```python
from build123d import *

# Parameters (mm, degrees)
RESSALTO_EXTRUS_O1_DEPTH   = 10
ESBO_O2_W                  = 6
ESBO_O2_H                  = 2.5
RESSALTO_EXTRUS_O2_DEPTH   = 8
ESBO_O3_W                  = 2.8
ESBO_O3_H                  = 2.8
CORTE_EXTRUS_O1_DEPTH      = 25.104680044
ESBO_O4_W                  = 6
ESBO_O4_H                  = 18
ESBO_O4_W_2                = 2.8
ESBO_O4_H_2                = 2.8
RESSALTO_EXTRUS_O3_DEPTH   = 2
CORTE_EXTRUS_O3_DEPTH      = 23.633727046
CORTE_EXTRUS_O3_DEPTH_BACK = 23.633727046
CORTE_EXTRUS_O4_DEPTH      = 24.796756081


with BuildPart() as part:
    # Esboço1 → Ressalto-extrusão1 (new body)
    with BuildSketch(Plane.XY):
        Polygon((-0.4, 0), (-0.57, 0), (-0.57, -2.5), (5.43, -2.5), (5.43, 0), (5.26, 0), (5.26, 10), (5.66, 11.25), (5.24, 12.5), (4.44, 12.5), (4.04, 11.25), (4.44, 10), (4.44, 0), (2.84, 0), (2.84, 10), (3.24, 11.25), (2.82, 12.5), (2.02, 12.5), (1.62, 11.25), (2.02, 10), (2.02, 0), (0.42, 0), (0.42, 10), (0.82, 11.25), (0.4, 12.5), (-0.4, 12.5), (-0.8, 11.25), (-0.4, 10), align=None)
    extrude(amount=RESSALTO_EXTRUS_O1_DEPTH)

    # Esboço2 → Ressalto-extrusão2 (add)
    with BuildSketch(Plane.XY.offset(10)):
        with Locations((2.43, -1.25)):
            Rectangle(ESBO_O2_W, ESBO_O2_H)
    extrude(amount=RESSALTO_EXTRUS_O2_DEPTH)

    # Esboço3 → Corte-extrusão1 (cut, through all)
    with BuildSketch(Plane.XZ.offset(2.5)):
        with Locations((2.43, 14)):
            Rectangle(ESBO_O3_W, ESBO_O3_H)
    extrude(amount=-CORTE_EXTRUS_O1_DEPTH, mode=Mode.SUBTRACT)

    # Esboço4 → Ressalto-extrusão3 (add)
    with BuildSketch(Plane.XZ.offset(2.5)):
        with Locations((2.43, 9)):
            Rectangle(ESBO_O4_W, ESBO_O4_H)
        with Locations((2.43, 14)):
            Rectangle(ESBO_O4_W_2, ESBO_O4_H_2, mode=Mode.SUBTRACT)
    extrude(amount=RESSALTO_EXTRUS_O3_DEPTH)

    # Esboço6 → Corte-extrusão3 (cut, two sides: drawn at the far end of the back side and taken through both)
    with BuildSketch(Plane(origin=(0, 0, 0), x_dir=(0, 0, -1), z_dir=(1, 0, 0)).offset(-CORTE_EXTRUS_O3_DEPTH_BACK)):
        Polygon((-18, 0), (-18, -2), (-14, -2), (-10.8, -2), (-10, 0), align=None)
    extrude(amount=CORTE_EXTRUS_O3_DEPTH + CORTE_EXTRUS_O3_DEPTH_BACK, mode=Mode.SUBTRACT)

    # Esboço7 → Corte-extrusão4 (cut, through all)
    with BuildSketch(Plane(origin=(0, -2, 0), x_dir=(1, 0, 0), z_dir=(0, 1, 0))):
        with BuildLine():
            Line((-0.57, -15.5), (-3.321312229, -15.5))
            Line((-3.321312229, -15.5), (-3.321312229, -18.857639181))
            Line((-3.321312229, -18.857639181), (8.546861735, -18.857639181))
            Line((8.546861735, -18.857639181), (8.546861735, -15.5))
            Line((8.546861735, -15.5), (5.43, -15.5))
            ThreePointArc((5.43, -15.5), (4.697766953, -17.267766953), (2.93, -18))
            Line((2.93, -18), (1.93, -18))
            ThreePointArc((1.93, -18), (0.162233047, -17.267766953), (-0.57, -15.5))
        make_face()
    extrude(amount=-CORTE_EXTRUS_O4_DEPTH, mode=Mode.SUBTRACT)


solid = part.part
```
The model under review builds one solid part; all positions refer to its coordinate system, in mm. A direction names the side the tool comes from. Round coordinates to 2 decimals unless told otherwise and drop trailing zeros. Loops run counter-clockwise (first coordinate to the right, second up) from the corner with the lowest first, then second, coordinate; pieces in that order, holes last. Notation, with made-up numbers: (40.5, 66.5) - (53.5, 66.5) arc R31 cw to (53.5, 101.5) - close; hole circle Ø1 at (64, -10). An arc over 180 degrees is marked (long way). Write each question's results on one line, items separated by ' | '. Start each with the question number.
Q1. Insertion check: P1, Ø3, axis at y = 8, z = 7.5, coming from the +X side; P2, Ø3, axis at y = -3.5, z = 14.5, coming from the +X side; P3, Ø3.5, axis at y = -2, z = 4, coming from the -X side; P4, Ø3, axis at x = 2.5, y = -3.5, coming from the -Z side. Each pin has a flat end and moves straight along its axis. Give the tip position at first contact, or say it passes through.
Q2. Take a section at A-A on z = 13.75. Give the boundary of the cut face in (x, y).
Q3. Wall thickness on line 1 along X through (y, z) = (6.5, 9.5); line 2 along X through (y, z) = (12.25, 4.5); line 3 along Z through (x, y) = (2.5, -2.5): over which ranges is each line inside the solid? List them lowest first. Write a range as [from, to].
Q4. Tool access review of faces 1 (the flat face through (2, -2, 16)), 2 (the flat face through (0.42, 5, 5)), 3 (the flat face through (0.6, 11.9, 4.9)), 4 (the flat face through (5.43, -2, 6)): name each direction out of +Z, -Z, +X, -X, +Y, -Y from which nothing blocks a thin tool from reaching the whole face with its end or side.
Q5. Take a section at D-D on y = -3.25. Give the boundary of the cut face in (x, z), plus the area to 3 significant figures.
Q6. Draft analysis for pull direction Z (two halves, no side actions). For faces 5 (the flat face through (-0.4, 5, 5)), 6 (the cylindrical face through (4.717, -3.232, 17.248)), 7 (the flat face through (1.03, -3, 14)), state which applies: pulls with the +Z half, pulls with the -Z half, needs draft (parallel to the pull), parting line crosses it, or undercut.
Q7. Take a section at B-B on y = 11. Give the boundary of the cut face in (x, z).
Q8. Take a section at C-C on x = 2.25. Give the boundary of the cut face in (y, z), plus the area to 3 significant figures.
Data:
1) P1: stops at x = 5.26 | P2: stops at x = 5.43 | P3: stops at x = -0.57 | P4: stops at z = 0
2) outline: (-0.57, -4.5) - (1.03, -4.5) - (1.03, -2) - (-0.57, -2) - close; (3.83, -4.5) - (5.43, -4.5) - (5.43, -2) - (3.83, -2) - close
3) line 1: x = [-0.4, 0.42], [2.02, 2.84], [4.44, 5.26] | line 2: x = [-0.48, 0.48], [1.94, 2.9], [4.36, 5.32] | line 3: z = [0, 12.6], [15.4, 18]
4) face 1: +Z, +X, -X, +Y | face 2: +Z, -Z | face 3: +Z, -Z, +Y | face 4: +Z, -Z, +X, -Y
5) outline: (-0.57, 0) - (5.43, 0) - (5.43, 15.5) arc R2.5 ccw to (2.93, 18) - (1.93, 18) arc R2.5 ccw to (-0.57, 15.5) - close; hole (1.03, 12.6) - (3.83, 12.6) - (3.83, 15.4) - (1.03, 15.4) - close | area: 97.5 mm²
6) face 5: needs draft | face 6: pulls with the +Z half | face 7: undercut
7) outline: (-0.72, 0) - (0.74, 0) - (0.74, 10) - (-0.72, 10) - close; (1.7, 0) - (3.16, 0) - (3.16, 10) - (1.7, 10) - close; (4.12, 0) - (5.58, 0) - (5.58, 10) - (4.12, 10) - close
8) outline: (-4.5, 0) - (12.5, 0) - (12.5, 10) - (0, 10) - (-2, 10.8) - (-2, 12.6) - (-4.5, 12.6) - close; (-4.5, 15.4) - (-2, 15.4) - (-2, 18) - (-4.5, 18) - close | area: 184 mm²
